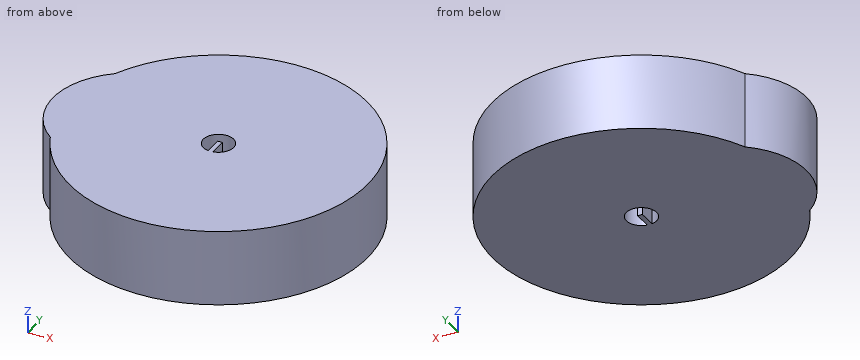
```python
from build123d import *

# Parameters (mm, degrees)
SKETCH_1_R          = 49
EXTRUDE_1_DEPTH     = 25
SKETCH_2_R          = 5
CUT_EXTRUDE_1_DEPTH = 25
SKETCH_3_W          = 1.555795937
SKETCH_3_H          = 6.849823777
EXTRUDE_4_DEPTH     = 25
EXTRUDE_5_DEPTH     = 25


with BuildPart() as part:
    # 草图1 → 凸台-拉伸1 (new body)
    with BuildSketch(Plane.XY):
        Circle(SKETCH_1_R)
    extrude(amount=EXTRUDE_1_DEPTH)

    # 草图2 → 切除-拉伸1 (cut)
    with BuildSketch(Plane(origin=(0, 0, 0), x_dir=(-1, 0, 0), z_dir=(0, 0, -1))):
        Circle(SKETCH_2_R)
    extrude(amount=-CUT_EXTRUDE_1_DEPTH, mode=Mode.SUBTRACT)

    # 草图3 → 凸台-拉伸4 (add)
    with BuildSketch(Plane(origin=(0, 0, 0), x_dir=(-1, 0, 0), z_dir=(0, 0, -1))):
        with Locations((0.010297919, -2.475862613)):
            Rectangle(SKETCH_3_W, SKETCH_3_H)
    extrude(amount=-EXTRUDE_4_DEPTH)

    # 草图7 → 凸台-拉伸5 (add)
    with BuildSketch(Plane(origin=(0, 0, 0), x_dir=(-1, 0, 0), z_dir=(0, 0, -1))):
        with BuildLine():
            ThreePointArc((44.732538493, 20), (54.385039322, 0), (44.732538493, -20))
            ThreePointArc((44.732538493, -20), (49, 0), (44.732538493, 20))
        make_face()
    extrude(amount=-EXTRUDE_5_DEPTH)


solid = part.part
```
Verification items for the finished model (mm, model axes). Coordinates: 2 decimals unless noted, no trailing zeros. Write each loop counter-clockwise with the first axis right and the second up, starting at its lowest first coordinate (ties: lowest second). Pieces come first, ordered by that corner, then holes. Notation, with made-up numbers: M -14,12.25 L 5,12.25 A9 ccw 5,20.25 Z; hole C 66.25,3 d11. An arc over 180 degrees is marked long. One line per item, written item: value.
Item 1: Section check B-B, the plane x = -29. Record the boundary of the cut face in (y, z), plus the area to 3 significant figures.
Check sheet entries:
outline: M -39.5,0 L 39.5,0 L 39.5,25 L -39.5,25 Z
area: 1,970 mm^2
Item 2: Section check C-C, the plane y = -17.5. Record the boundary of the cut face in (x, z), plus the area to 3 significant figures.
Check sheet entries:
outline: M -47.45,0 L 45.77,0 L 45.77,25 L -47.45,25 Z
area: 2,330 mm^2
Item 3: Scan lines: line 1 along Y through (x, z) = (0, 7); line 2 along Y through (x, z) = (41.5, 6.25); line 3 along Y through (x, z) = (-27, 13.5). Record each from-to range of solid material in increasing order.
Check sheet entries:
line 1: y = -49 to 0.95, 5 to 49
line 2: y = -26.05 to 26.05
line 3: y = -40.89 to 40.89
Item 4: Gauge pin test, flat ends, axial feed: pin 1 Ø8 at (x, z) = (22.5, 9.5) entering from +Y; pin 2 Ø8 at (y, z) = (37, 12.5) entering from +X; pin 3 Ø1.8 at (y, z) = (-1.5, 16.5) entering from +X. Record the tip position at first contact, or that the pin passes through.
Check sheet entries:
pin 1: stops at y = 45.37
pin 2: stops at x = 36.22
pin 3: stops at x = 49
Item 5: Section check A-A, the plane z = 15.5. Record the boundary of the cut face in (x, y).
Check sheet entries:
outline: M -44.73,-20 A49 ccw long -44.73,20 A25.55 ccw Z; hole M -0.79,-4.94 L -0.79,0.95 L 0.77,0.95 L 0.77,-4.94 A5 ccw long Z
